```python
from build123d import *

# Parameters (mm, degrees)
SKETCH2_R           = 8.5
BOSS_EXTRUDE1_DEPTH = 10
SKETCH3_R           = 11.175
CUT_EXTRUDE1_DEPTH  = 7
SKETCH4_W           = 70
SKETCH4_H           = 5
BOSS_EXTRUDE3_DEPTH = 20
SKETCH5_R           = 1.64
CUT_EXTRUDE2_DEPTH  = 20
CHAMFER1_SIZE       = 0.4
CHAMFER3_SIZE       = 0.4
BOSS_EXTRUDE4_DEPTH = 5.4
BOSS_EXTRUDE5_DEPTH = 5


with BuildPart() as part:
    # Sketch2 → Boss-Extrude1 (new body)
    with BuildSketch(Plane.XY):
        with BuildLine():
            Line((0, 0), (-70, 0))
            Line((-70, 0), (-70, 115))
            ThreePointArc((-70, 115), (-65.606601718, 125.606601718), (-55, 130))
            Line((-55, 130), (-15, 130))
            ThreePointArc((-15, 130), (-4.393398282, 125.606601718), (0, 115))
            Line((0, 115), (0, 0))
        make_face()
        with Locations((-35, 108)):
            Circle(SKETCH2_R, mode=Mode.SUBTRACT)
    extrude(amount=BOSS_EXTRUDE1_DEPTH)

    # Sketch3 → Cut-Extrude1 (cut)
    with BuildSketch(Plane.XY.offset(10)):
        with Locations((-35, 108)):
            Circle(SKETCH3_R)
    extrude(amount=-CUT_EXTRUDE1_DEPTH, mode=Mode.SUBTRACT)

    # Sketch4 → Boss-Extrude3 (add)
    with BuildSketch(Plane.XY.offset(10)):
        with Locations((-35, 2.5)):
            Rectangle(SKETCH4_W, SKETCH4_H)
    extrude(amount=BOSS_EXTRUDE3_DEPTH)

    # Sketch5 → Cut-Extrude2 (cut)
    with BuildSketch(Plane(origin=(0, 5, 0), x_dir=(1, 0, 0), z_dir=(0, 1, 0))):
        with Locations(Location((-60, -18, 0), (0, 0, 270))):
            Circle(SKETCH5_R)
        with Locations(Location((-35, -24, 0), (0, 0, 270))):
            Circle(SKETCH5_R)
        with Locations(Location((-10, -18, 0), (0, 0, 270))):
            Circle(SKETCH5_R)
    extrude(amount=-CUT_EXTRUDE2_DEPTH, mode=Mode.SUBTRACT)

    # Chamfer1
    chamfer1_edges = [part.edges().sort_by_distance(p)[0] for p in [
        (-35, 5, 22.36),
    ]]
    chamfer(chamfer1_edges, length=CHAMFER1_SIZE)

    # Chamfer3
    chamfer3_edges = [part.edges().sort_by_distance(p)[0] for p in [
        (-60, 5, 16.36),
        (-10, 5, 16.36),
    ]]
    chamfer(chamfer3_edges, length=CHAMFER3_SIZE)

    # Sketch6 → Boss-Extrude4 (add)
    with BuildSketch(Plane.XY.offset(10)):
        with BuildLine():
            Line((-21, 90.5), (-23.5, 90.5))
            ThreePointArc((-23.5, 90.5), (-35, 79), (-46.5, 90.5))
            Line((-46.5, 90.5), (-49, 90.5))
            ThreePointArc((-49, 90.5), (-35, 76.5), (-21, 90.5))
        make_face()
    extrude(amount=BOSS_EXTRUDE4_DEPTH)

    # Sketch7 → Boss-Extrude5 (add)
    with BuildSketch(Plane.XY.offset(15.4)):
        with BuildLine():
            ThreePointArc((-23.5, 90.5), (-35, 79), (-46.5, 90.5))
            Line((-46.5, 90.5), (-49, 90.5))
            ThreePointArc((-49, 90.5), (-35, 76.5), (-21, 90.5))
            Line((-21, 90.5), (-23.5, 90.5))
        make_face()
        with BuildLine():
            Line((-40.125, 90.5), (-46.5, 90.5))
            ThreePointArc((-46.5, 90.5), (-35, 79), (-23.5, 90.5))
            Line((-23.5, 90.5), (-29.875, 90.5))
            ThreePointArc((-29.875, 90.5), (-30.027261821, 89.260040323), (-30.475, 88.093758117))
            Line((-30.475, 88.093758117), (-30.475, 85.375))
            Line((-30.475, 85.375), (-35, 85.375))
            Line((-35, 85.375), (-39.525, 85.375))
            Line((-39.525, 85.375), (-39.525, 88.093758117))
            ThreePointArc((-39.525, 88.093758117), (-39.972738179, 89.260040323), (-40.125, 90.5))
        make_face()
        with BuildLine():
            ThreePointArc((-48.934070004, 91.857089942), (-48.983507787, 91.17934525), (-49, 90.5))
            Line((-49, 90.5), (-46.5, 90.5))
            Line((-46.5, 90.5), (-40.125, 90.5))
            Line((-40.125, 90.5), (-40.125, 92.5))
            Line((-40.125, 92.5), (-48, 92.5))
            ThreePointArc((-48, 92.5), (-48.566970042, 92.323738412), (-48.934070004, 91.857089942))
        make_face()
        with BuildLine():
            Line((-23.5, 90.5), (-21, 90.5))
            ThreePointArc((-21, 90.5), (-21.016492213, 91.17934525), (-21.065929996, 91.857089942))
            ThreePointArc((-21.065929996, 91.857089942), (-21.433029958, 92.323738412), (-22, 92.5))
            Line((-22, 92.5), (-29.875, 92.5))
            Line((-29.875, 92.5), (-29.875, 90.5))
            Line((-29.875, 90.5), (-23.5, 90.5))
        make_face()
    extrude(amount=BOSS_EXTRUDE5_DEPTH)


solid = part.part
```
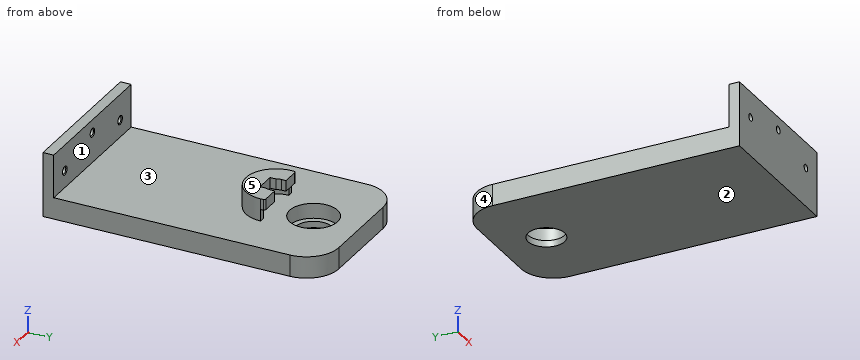
Can you work these out from the model? Positions are in its coordinate system, mm. Face numbers are marked on the shaded views. A direction names the side the tool comes from. Round coordinates to 2 decimals unless told otherwise and drop trailing zeros. Loops run counter-clockwise (first coordinate to the right, second up) from the corner with the lowest first, then second, coordinate; pieces in that order, holes last. Notation, with made-up numbers: M -22.5,-35 L 31.5,-35 A17 cw 31.5,-29 Z; hole C 32,59 d4. An arc over 180 degrees is marked long. Write item = value, one per line. Start each with the question number.
(1) Suppose I cut it at C-C on z = 24. Write out the boundary of the cut face in (x, y), plus the area to 3 significant figures.
(2) I need wall thicknesses on line 1 along X through (y, z) = (108, 1.5); line 2 along Y through (x, z) = (-35, 2.25); line 3 along Z through (x, y) = (-66.5, 51). Which ranges of each line are inside material? Lowest first, please.
(3) Which directions (+Z, -Z, +X, -X, +Y, -Y) give clear straight access to the entire face, cutting with the end or side of a thin tool? Please do the marked faces 1 and 2.
(4) Suppose I cut it at D-D on x = -60. Write out the boundary of the cut face in (y, z), plus the area to 3 significant figures.
(5) I'm going to push flat-ended pins straight in: P1, Ø2.5, axis at x = -44, z = 17, coming from the +Y side; P2, Ø8, axis at x = -29, y = 81, coming from the +Z side; P3, Ø3, axis at y = 86.5, z = 17.5, coming from the +X side (3 decimals). Where does each tip first touch, or does it pass through?
(6) Suppose I cut it at A-A on z = 18. Write out the boundary of the cut face in (x, y) (3 decimals).
(7) Suppose I cut it at B-B on y = 108. Write out the boundary of the cut face in (x, z) (3 decimals), plus the area to 3 significant figures.
(8) If we mould it in two halves opening along Y, with no side actions, what happens to the marked faces 3, 4 and 5? For each: released by +Y, released by -Y, zero draft, split by the parting line, or undercut.
Answer block:
q1.outline = M -70,0 L -36.64,0 L -36.64,4.6 L -37.04,5 L -70,5 Z; M -33.36,0 L 0,0 L 0,5 L -32.96,5 L -33.36,4.6 Z
q1.area = 333 mm²
q2.line_1 = -70 to -43.5, -26.5 to 0
q2.line_2 = 0 to 99.5, 116.5 to 130
q2.line_3 = 0 to 10
q3.face_1 = +Z, +X, -X
q3.face_2 = -Z, +X, -X, +Y, -Y
q4.outline = M 0,0 L 129.14,0 L 129.14,10 L 5,10 L 5,15.96 L 4.6,16.36 L 0,16.36 Z; M 0,19.64 L 4.6,19.64 L 5,20.04 L 5,30 L 0,30 Z
q4.area = 1,370 mm²
q5.P1 = 92.5
q5.P2 = 20.4
q5.P3 = -21.225
q6.outline = M -70,0 L -61.64,0 L -61.64,4.6 L -62.04,5 L -70,5 Z; M -58.36,0 L -11.64,0 L -11.64,4.6 L -12.04,5 L -57.96,5 L -58.36,4.6 Z; M -48.934,91.857 A14 ccw long -21.066,91.857 A1 ccw -22,92.5 L -29.875,92.5 L -29.875,90.5 A5.125 cw -30.475,88.094 L -30.475,85.375 L -39.525,85.375 L -39.525,88.094 A5.125 cw -40.125,90.5 L -40.125,92.5 L -48,92.5 A1 ccw Z; M -8.36,0 L 0,0 L 0,5 L -7.96,5 L -8.36,4.6 Z
q7.outline = M -70,0 L -43.5,0 L -43.5,3 L -46.175,3 L -46.175,10 L -70,10 Z; M -26.5,0 L 0,0 L 0,10 L -23.825,10 L -23.825,3 L -26.5,3 Z
q7.area = 493 mm²
q8.face_3 = undercut
q8.face_4 = released by +Y
q8.face_5 = zero draft
